Design review of the part built by this model. Coordinates are the model's own, in mm. A direction names the side the tool comes from. Give positions to 0.01 mm unless a question says otherwise; leave off trailing zeros. Order: outer loops, then holes, each group sorted by start corner. A loop starts at its lowest first (then second) coordinate and runs counter-clockwise, first axis right, second up. Notation, with made-up numbers: (56, -6) -> (76, -6) arc R32 ccw to (76, 25) -> close; hole circle Ø9 at (31.25, 31). An arc over 180 degrees is marked (long way). One line per item, written item: value.
from build123d import *

# Parameters (mm, degrees)
SKETCH1_R          = 1.3
EXTRUDE1_DEPTH     = 21.5
EXTRUDE2_DEPTH     = 1.2
FILLET1_R          = 0.5
SKETCH4_W          = 11.5
SKETCH4_H          = 26.1
CUT_EXTRUDE2_DEPTH = 13.2
CUT_EXTRUDE3_DEPTH = 3
CUT_EXTRUDE4_START = -13.2
CUT_EXTRUDE4_DEPTH = 13.2
SKETCH6_R          = 3.3
CUT_EXTRUDE5_DEPTH = 46.164504919


with BuildPart() as part:
    # Sketch1 → Extrude1 (new body)
    with BuildSketch(Plane(origin=(0, 0, 0), x_dir=(1, 0, 0), z_dir=(0, 1, 0))):
        with BuildLine():
            Line((-34.5, 13.05), (6.5, 13.05))
            ThreePointArc((6.5, 13.05), (10.035533906, 11.585533906), (11.5, 8.05))
            Line((11.5, 8.05), (11.5, -8.05))
            ThreePointArc((11.5, -8.05), (10.035533906, -11.585533906), (6.5, -13.05))
            Line((6.5, -13.05), (-34.5, -13.05))
            ThreePointArc((-34.5, -13.05), (-35.207106781, -12.757106781), (-35.5, -12.05))
            Line((-35.5, -12.05), (-35.5, -5.8))
            Line((-35.5, -5.8), (-36.8, -5.8))
            Line((-36.8, -5.8), (-36.8, 5.8))
            Line((-36.8, 5.8), (-35.5, 5.8))
            Line((-35.5, 5.8), (-35.5, 12.05))
            ThreePointArc((-35.5, 12.05), (-35.207106781, 12.757106781), (-34.5, 13.05))
        make_face()
        with Locations(Location((-31.8, 9.2, 0), (0, 0, 270))):
            Circle(SKETCH1_R, mode=Mode.SUBTRACT)
        with Locations(Location((8.5, 9, 0), (0, 0, 270))):
            Circle(SKETCH1_R, mode=Mode.SUBTRACT)
        with Locations(Location((8.5, -9, 0), (0, 0, 90))):
            Circle(SKETCH1_R, mode=Mode.SUBTRACT)
        with Locations(Location((-31.8, -9.2, 0), (0, 0, 90))):
            Circle(SKETCH1_R, mode=Mode.SUBTRACT)
    extrude(amount=EXTRUDE1_DEPTH)

    # Sketch2 → Extrude2 (add)
    with BuildSketch(Plane(origin=(0, 21.5, 0), x_dir=(-1, 0, 0), z_dir=(0, 1, 0))):
        with BuildLine():
            Line((33.000666235, -7.121923824), (34.111271501, -5.199722402))
            ThreePointArc((34.111271501, -5.199722402), (34.477275392, -4.833894464), (34.977136574, -4.7))
            Line((34.977136574, -4.7), (35.7, -4.7))
            Line((35.7, -4.7), (35.7, 4.7))
            Line((35.7, 4.7), (34.977136574, 4.7))
            ThreePointArc((34.977136574, 4.7), (34.477275392, 4.833894464), (34.111271501, 5.199722402))
            Line((34.111271501, 5.199722402), (33.000666235, 7.121923824))
            ThreePointArc((33.000666235, 7.121923824), (30.488773811, 7.189854264), (29.414271687, 9.461343485))
            ThreePointArc((29.414271687, 9.461343485), (16.6, 0), (29.414271687, -9.461343485))
            ThreePointArc((29.414271687, -9.461343485), (30.488773811, -7.189854264), (33.000666235, -7.121923824))
        make_face()
    extrude(amount=EXTRUDE2_DEPTH)

    # Fillet1
    fillet1_edges = [part.edges().sort_by_distance(p)[0] for p in [
        (-30.488773811, 22.7, 7.189854264),
        (-16.6, 22.7, 0),
        (-30.488773811, 22.7, -7.189854264),
        (-33.555968868, 22.7, -6.160823113),
        (-34.477275392, 22.7, -4.833894464),
        (-35.338568287, 22.7, -4.7),
        (-35.7, 22.7, 0),
        (-35.338568287, 22.7, 4.7),
        (-34.477275392, 22.7, 4.833894464),
        (-33.555968868, 22.7, 6.160823113),
    ]]
    fillet(fillet1_edges, radius=FILLET1_R)

    # Sketch4 → Cut-Extrude2 (cut)
    with BuildSketch(Plane(origin=(0, 21.5, 0), x_dir=(-1, 0, 0), z_dir=(0, 1, 0))):
        with Locations((-5.75, 0)):
            Rectangle(SKETCH4_W, SKETCH4_H)
    extrude(amount=-CUT_EXTRUDE2_DEPTH, mode=Mode.SUBTRACT)

    # Sketch5 → Cut-Extrude3 (cut)
    with BuildSketch(Plane.XZ):
        with BuildLine():
            Line((-3.5, -13.05), (-3.5, 13.05))
            Line((-3.5, 13.05), (6.5, 13.05))
            ThreePointArc((6.5, 13.05), (10.035533906, 11.585533906), (11.5, 8.05))
            Line((11.5, 8.05), (11.5, -8.05))
            ThreePointArc((11.5, -8.05), (10.035533906, -11.585533906), (6.5, -13.05))
            Line((6.5, -13.05), (-3.5, -13.05))
        make_face()
    extrude(amount=-CUT_EXTRUDE3_DEPTH, mode=Mode.SUBTRACT)

    # Sketch3 → Cut-Extrude4 (cut)
    with BuildSketch(Plane(origin=(0, 21.5, 0), x_dir=(-1, 0, 0), z_dir=(0, 1, 0)).offset(CUT_EXTRUDE4_START)):
        with BuildLine():
            Line((20.7, 8.023091673), (20.7, 11.75))
            Line((20.7, 11.75), (-6.5, 11.75))
            ThreePointArc((-6.5, 11.75), (-7.422418806, 11.633175065), (-8.286588144, 11.290077592))
            ThreePointArc((-8.286588144, 11.290077592), (-6.441484419, 7.974079144), (-10.2, 7.450806662))
            Line((-10.2, 7.450806662), (-10.2, -7.450806662))
            ThreePointArc((-10.2, -7.450806662), (-6.441484419, -7.974079144), (-8.286588144, -11.290077592))
            ThreePointArc((-8.286588144, -11.290077592), (-7.422418806, -11.633175065), (-6.5, -11.75))
            Line((-6.5, -11.75), (20.7, -11.75))
            Line((20.7, -11.75), (20.7, -8.023091673))
            ThreePointArc((20.7, -8.023091673), (16.6, 0), (20.7, 8.023091673))
        make_face()
    extrude(amount=CUT_EXTRUDE4_DEPTH, mode=Mode.SUBTRACT)

    # Sketch6 → Cut-Extrude5 (cut, through all)
    with BuildSketch(Plane.XZ):
        with Locations(Location((0, 0, 0), (0, 0, 270))):
            Circle(SKETCH6_R)
    extrude(amount=-CUT_EXTRUDE5_DEPTH, mode=Mode.SUBTRACT)


solid = part.part
Item 1: Clearance check with flat-ended pins moving along their axes: P1, Ø6, axis at x = 5, z = 2, coming from the -Y side; P2, Ø2, axis at y = 10.5, z = 4.5, coming from the +X side; P3, Ø1.9, axis at y = 12.5, z = 10.5, coming from the +X side; P4, Ø1.5, axis at x = -20, z = 1.5, coming from the -Y side. State where each tip first meets the part, or that it passes through.
Returned:
P1: y = 3
P2: x = -17.24
P3: x = -20.7
P4: y = 0
Item 2: Add section B-B on y = 12.5. Give the boundary of the cut face in (x, z), plus the area to 3 significant figures.
Returned:
outline: (-36.8, -5.8) -> (-35.5, -5.8) -> (-35.5, -12.05) arc R1 ccw to (-34.5, -13.05) -> (0, -13.05) -> (0, -11.75) -> (-20.7, -11.75) -> (-20.7, -8.02) arc R9.9 ccw to (-20.7, 8.02) -> (-20.7, 11.75) -> (0, 11.75) -> (0, 13.05) -> (-34.5, 13.05) arc R1 ccw to (-35.5, 12.05) -> (-35.5, 5.8) -> (-36.8, 5.8) -> close; hole circle Ø2.6 at (-31.8, -9.2); hole circle Ø2.6 at (-31.8, 9.2)
area: 490 mm²
Item 3: Add section A-A on z = 0. Give the boundary of the cut face in (x, y), plus the area to 3 significant figures.
Returned:
outline: (-36.8, 0) -> (-3.5, 0) -> (-3.5, 3) -> (-3.3, 3) -> (-3.3, 8.3) -> (-16.6, 8.3) -> (-16.6, 22.2) arc R0.5 ccw to (-17.1, 22.7) -> (-35.2, 22.7) arc R0.5 ccw to (-35.7, 22.2) -> (-35.7, 21.5) -> (-36.8, 21.5) -> close; (3.3, 3) -> (11.5, 3) -> (11.5, 8.3) -> (3.3, 8.3) -> close
area: 610 mm²
Item 4: To check wall thickness, follow line 1 along X through (y, z) = (5.8, -9); line 2 along X through (y, z) = (7.5, -8.5); line 3 along Z through (x, y) = (-1.5, 14). State the ranges of each line that lie inside material, in increasing order. Write a range as from..to.
Returned:
line 1: -35.5..-33.08, -30.52..7.2, 9.8..11.41
line 2: -35.5..-32.9, -30.7..7.3, 9.7..11.48
line 3: -13.05..-11.75, 11.75..13.05
Item 5: Draft analysis for pull direction X (two halves, no side actions). For faces 4 (the flat face through (-36.8, 11, 0)), 5 (the flat face through (0, 15, -12)), 6 (the cylindrical face through (-30.52, 21.85, 7.17)), state which applies: pulls with the +X half, pulls with the -X half, needs draft (parallel to the pull), parting line crosses it, or undercut.
Returned:
face 4: pulls with the -X half
face 5: pulls with the +X half
face 6: undercut
Item 6: Machinability: for faces 1 (the flat face through (-10, 15, -11.75)), 2 (the flat face through (-36, 11, -5.8)), 3 (the flat face through (-36, 11, 5.8)), which of the approach directions +Z, -Z, +X, -X, +Y, -Y give a long, thin tool a straight path to every point of the face, cutting with its end or side? Answer none if there is none.
Returned:
face 1: +X, +Y
face 2: -Z, -X, +Y, -Y
face 3: +Z, -X, +Y, -Y
Item 7: Add section C-C on x = 8.5. Give the boundary of the cut face in (y, z).
Returned:
outline: (3, -12.63) -> (8.3, -12.63) -> (8.3, -10.3) -> (3, -10.3) -> close; (3, -7.7) -> (8.3, -7.7) -> (8.3, 7.7) -> (3, 7.7) -> close; (3, 10.3) -> (8.3, 10.3) -> (8.3, 12.63) -> (3, 12.63) -> close
Item 8: Add section D-D on y = 6.5. Give the boundary of the cut face in (x, z).
Returned:
outline: (-36.8, -5.8) -> (-35.5, -5.8) -> (-35.5, -12.05) arc R1 ccw to (-34.5, -13.05) -> (6.5, -13.05) arc R5 ccw to (11.5, -8.05) -> (11.5, 8.05) arc R5 ccw to (6.5, 13.05) -> (-34.5, 13.05) arc R1 ccw to (-35.5, 12.05) -> (-35.5, 5.8) -> (-36.8, 5.8) -> close; hole circle Ø2.6 at (-31.8, -9.2); hole circle Ø2.6 at (-31.8, 9.2); hole circle Ø6.6 at (0, 0); hole circle Ø2.6 at (8.5, -9); hole circle Ø2.6 at (8.5, 9)
